Geometry check sheet. Reference: the model listing, model coordinates, mm. Give positions to 0.01 mm unless a question says otherwise; leave off trailing zeros. Write each loop counter-clockwise with the first axis right and the second up, starting at its lowest first coordinate (ties: lowest second). Pieces come first, ordered by that corner, then holes. Notation, with made-up numbers: (-38.75, -13.5) -> (18.25, -13.5) arc R24 ccw to (18.25, 23.5) -> close; hole circle Ø2 at (26, 66.25). An arc over 180 degrees is marked (long way). Write item = value, one per line. Start each with the question number.
1. Thickness scan on line 1 along X through (y, z) = (1.2, 125.5); line 2 along X through (y, z) = (2.15, 300); line 3 along X through (y, z) = (0.6, -252.5). Record the ranges inside material, lowest first.
2. Depth check by flat-ended pin: P1, Ø1.5, axis at x = 341, y = 1, coming from the -Z side; P2, Ø3, axis at x = 35, z = 240, coming from the -Y side; P3, Ø1.5, axis at y = 1, z = -215, coming from the +X side; P4, Ø1.5, axis at y = 2, z = 171.5, coming from the -X side. Enter the tip coordinate at first touch or a pass-through.
3. Cross-section at B-B, the plane z = -229. Record the cut outline in (x, y).
4. Cross-section at C-C, the plane x = 261. Record the cut outline in (y, z).
5. Cross-section at A-A, the plane y = 0.45. Record the cut outline in (x, z).
```python
from build123d import *

# Parameters (mm, degrees)
BASE_DEPTH         = 3
SKETCH2_R          = 2.5
CUT_EXTRUDE2_DEPTH = 495.98383812


with BuildPart() as part:
    # Sketch1 → Base (new body)
    with BuildSketch(Plane(origin=(0, 0, 0), x_dir=(1, 0, 0), z_dir=(0, 1, 0))):
        Polygon((-350, -130), (-328, -130), (-328, -108), (-130, -108), (-130, -130), (-130, -350), (130, -350), (130, -130), (130, -108), (328, -108), (328, -130), (350, -130), (350, 130), (328, 130), (328, 108), (130, 108), (130, 130), (130, 350), (-130, 350), (-130, 130), (-130, 108), (-328, 108), (-328, 130), (-350, 130), align=None)
    extrude(amount=BASE_DEPTH)

    # Sketch2 → Cut-Extrude2 (cut, through all)
    with BuildSketch(Plane.XZ):
        with Locations(Location((-25, 300, 0), (0, 0, 270))):
            Circle(SKETCH2_R)
        with Locations(Location((35, 300, 0), (0, 0, 270))):
            Circle(SKETCH2_R)
        with Locations(Location((-25, 240, 0), (0, 0, 270))):
            Circle(SKETCH2_R)
        with Locations(Location((35, 240, 0), (0, 0, 270))):
            Circle(SKETCH2_R)
    extrude(amount=-CUT_EXTRUDE2_DEPTH, mode=Mode.SUBTRACT)


solid = part.part
```
Answers:
q1.line_1 = -350 to -328, -130 to 130, 328 to 350
q1.line_2 = -130 to -27.5, -22.5 to 32.5, 37.5 to 130
q1.line_3 = -130 to 130
q2.P1 = -130
q2.P2 = through
q2.P3 = 130
q2.P4 = -130
q3.outline = (-130, 0) -> (130, 0) -> (130, 3) -> (-130, 3) -> close
q4.outline = (0, -108) -> (3, -108) -> (3, 108) -> (0, 108) -> close
q5.outline = (-350, -130) -> (-328, -130) -> (-328, -108) -> (-130, -108) -> (-130, -350) -> (130, -350) -> (130, -108) -> (328, -108) -> (328, -130) -> (350, -130) -> (350, 130) -> (328, 130) -> (328, 108) -> (130, 108) -> (130, 350) -> (-130, 350) -> (-130, 108) -> (-328, 108) -> (-328, 130) -> (-350, 130) -> close; hole circle Ø5 at (-25, 240); hole circle Ø5 at (-25, 300); hole circle Ø5 at (35, 240); hole circle Ø5 at (35, 300)
